Build history of the part. All positions in model axes, mm. A direction names the side the tool comes from. Coordinates: 2 decimals unless noted, no trailing zeros. Loops run counter-clockwise (first coordinate to the right, second up) from the corner with the lowest first, then second, coordinate; pieces in that order, holes last. Notation, with made-up numbers: (-13, -6) - (15, -6) arc R24 ccw to (15, 6) - close; hole circle Ø10 at (-2.75, 61.25). An arc over 180 degrees is marked (long way). One line per item, written item: value.
```python
from build123d import *

# Parameters (mm, degrees)
F0_R     = 9.525
F1_DEPTH = 12.7
F0_W     = 12.7
F0_H     = 50.8
F2_DEPTH = 25.4
F6_SIZE2 = 2.54
F6_SIZE  = 2.54


with BuildPart() as f1:
    # F0 (on Front) → F1 (new body, symmetric)
    with BuildSketch(Plane.XZ):
        with BuildLine():
            Line((-50.8, 0), (-12.7, 0))
            Line((-12.7, 0), (-12.7, 50.8))
            Line((-12.7, 50.8), (-50.8, 50.8))
            ThreePointArc((-50.8, 50.8), (-76.2, 25.4), (-50.8, 0))
        make_face()
        with Locations((-50.8, 25.4)):
            Circle(F0_R, mode=Mode.SUBTRACT)
    extrude(amount=F1_DEPTH, both=True)

    # F0 (on Front) → F2 (join, symmetric)
    with BuildSketch(Plane.XZ):
        with Locations((-6.35, 25.4)):
            Rectangle(F0_W, F0_H)
    extrude(amount=F2_DEPTH, both=True)

    # F4 (on Front) → F5 (revolve)
    with BuildSketch(Plane.XZ):
        with BuildLine():
            Line((0, 41.91), (0, 25.4))
            Line((0, 25.4), (76.2, 25.4))
            Line((76.2, 25.4), (76.2, 38.1))
            Line((76.2, 38.1), (3.81, 38.1))
            ThreePointArc((3.81, 38.1), (1.1159231637, 39.2159231637), (0, 41.91))
        make_face()
    revolve(axis=Axis((44.0839976072, 0, 25.4), (1, 0, 0)))

    # F6
    f6_edges = [f1.edges().sort_by_distance(p)[0] for p in [
        (76.2, 0, 12.7),
    ]]
    chamfer(f6_edges, length=F6_SIZE, length2=F6_SIZE2)


solid = f1.part
```
Item 1: Probe probe 1 along Z at (x, y) = (-50, -6); probe 2 along Y at (x, z) = (5, 25); probe 3 along X at (y, z) = (17.5, 5). List the from-to ranges inside material, lowest first. Write a range as from..to.
Check result:
probe 1: z = 0..15.91, 34.89..50.8
probe 2: y = -12.69..12.69
probe 3: x = -12.7..0
Item 2: Cut at A-A, the plane y = 0. Write the cut outline in (x, z) (3 decimals), then the cut area to 3 significant figures.
Check result:
outline: (-50.8, 0) - (0, 0) - (0, 8.89) arc R3.81 cw to (3.81, 12.7) - (73.66, 12.7) - (76.2, 15.24) - (76.2, 35.56) - (73.66, 38.1) - (3.81, 38.1) arc R3.81 cw to (0, 41.91) - (0, 50.8) - (-50.8, 50.8) arc R25.4 ccw to start; hole circle Ø19.05 at (-50.8, 25.4)
area: 5,240 mm^2
Item 3: Drop flat-ended pins along their axis: P1, Ø2, axis at x = -6, y = -20, coming from the -Z side; P2, Ø4, axis at x = 48.5, y = 16, coming from the +Z side; P3, Ø5, axis at x = -42.5, z = 34, coming from the -Y side; P4, Ø1.5, axis at x = -54, y = -2.5, coming from the -Z side. Give the stop position or say it passes through.
Check result:
P1: stops at z = 0
P2: passes through
P3: stops at y = -12.7
P4: stops at z = 0.12
Item 4: Tool access for faces 1 (the face through (0, -17, 25)), 2 (the face through (-38, 12.7, 26)), 3 (the face through (-38, -12.7, 26)): list every direction of +Z, -Z, +X, -X, +Y, -Y with a clear straight run to the whole face (end or side of a thin tool).
Check result:
face 1: +X
face 2: +Z, -Z, -X, +Y
face 3: +Z, -Z, -X, -Y
Item 5: Pull direction X, two halves, no side cores. Call faces 4 (the face through (76.2, 0, 26)), 5 (the face through (-12.7, 19, 25)), 6 (the face through (-46.4, 0.18, 16.95)), 7 (the face through (-20, 0, 50.8)): released by +X, released by -X, zero draft, split by the parting line, or undercut.
Check result:
face 4: released by +X
face 5: released by -X
face 6: undercut
face 7: zero draft
Item 6: Cut at D-D, the plane x = 46. Write the cut outline in (y, z).
Check result:
outline: circle Ø25.4 at (0, 25.4)
Item 7: Cut at C-C, the plane x = -28. Write the cut outline in (y, z), then the cut area to 3 significant figures.
Check result:
outline: (-12.7, 0) - (12.7, 0) - (12.7, 50.8) - (-12.7, 50.8) - close
area: 1,290 mm^2
Item 8: Cut at B-B, the plane z = 25.4. Write the cut outline in (x, y) (3 decimals).
Check result:
outline: (-76.2, -12.7) - (-60.325, -12.7) - (-60.325, 12.7) - (-76.2, 12.7) - close; (-41.275, -12.7) - (-12.7, -12.7) - (-12.7, -25.4) - (0, -25.4) - (0, -16.51) arc R3.81 cw to (3.81, -12.7) - (73.66, -12.7) - (76.2, -10.16) - (76.2, 10.16) - (73.66, 12.7) - (3.81, 12.7) arc R3.81 cw to (0, 16.51) - (0, 25.4) - (-12.7, 25.4) - (-12.7, 12.7) - (-41.275, 12.7) - close
